Input: dimensioned drawing with shaded views. Units: mm. Origin: part minimum x, y, z. Round coordinates to 2 decimals unless told otherwise and drop trailing zeros. Loops run counter-clockwise (first coordinate to the right, second up) from the corner with the lowest first, then second, coordinate; pieces in that order, holes last. Notation, with made-up numbers: M -13.75,62.25 L 29.25,62.25 A23 ccw 29.25,99.25 Z; hole C 64.25,87 d11. An arc over 180 degrees is marked long. Write each question's results on one line, items separated by ' | '. Start each with the question number.
1. Draft query along Z for the marked faces 1, 2, 3 and 4. Return one class per face: released by +Z, released by -Z, zero draft, split by the parting line, or undercut.
2. Ray query, line 1 (Y direction, x = 4.65, z = 17.5); line 2 (Y direction, x = 4.35, z = 24); line 3 (X direction, y = 15.5, z = 9.25). Return the intervals inside material, ascending.
3. Contact query for flat-ended pins moving along their axis: pin 1 Ø7.5 at (y, z) = (12.37, 17.5) entering from -X; pin 2 Ø2 at (x, z) = (4.5, 18.5) entering from -Y; pin 3 Ø4 at (y, z) = (14.5, 23.5) entering from -X; pin 4 Ø2 at (x, z) = (1.5, 10.5) entering from +Y. Output: stop coordinate, or through.
4. Section A-A on z = 14.25. Output: boundary loops of the cut face in (x, y) (1 decimal), and give its area (3 significant figures).
5. Section C-C on x = 1.65. Output: boundary loops of the cut face in (y, z) (1 decimal).
6. Section D-D on z = 17.5. Output: boundary loops of the cut face in (x, y).
7. Section B-B on y = 11.5. Output: boundary loops of the cut face in (x, z).
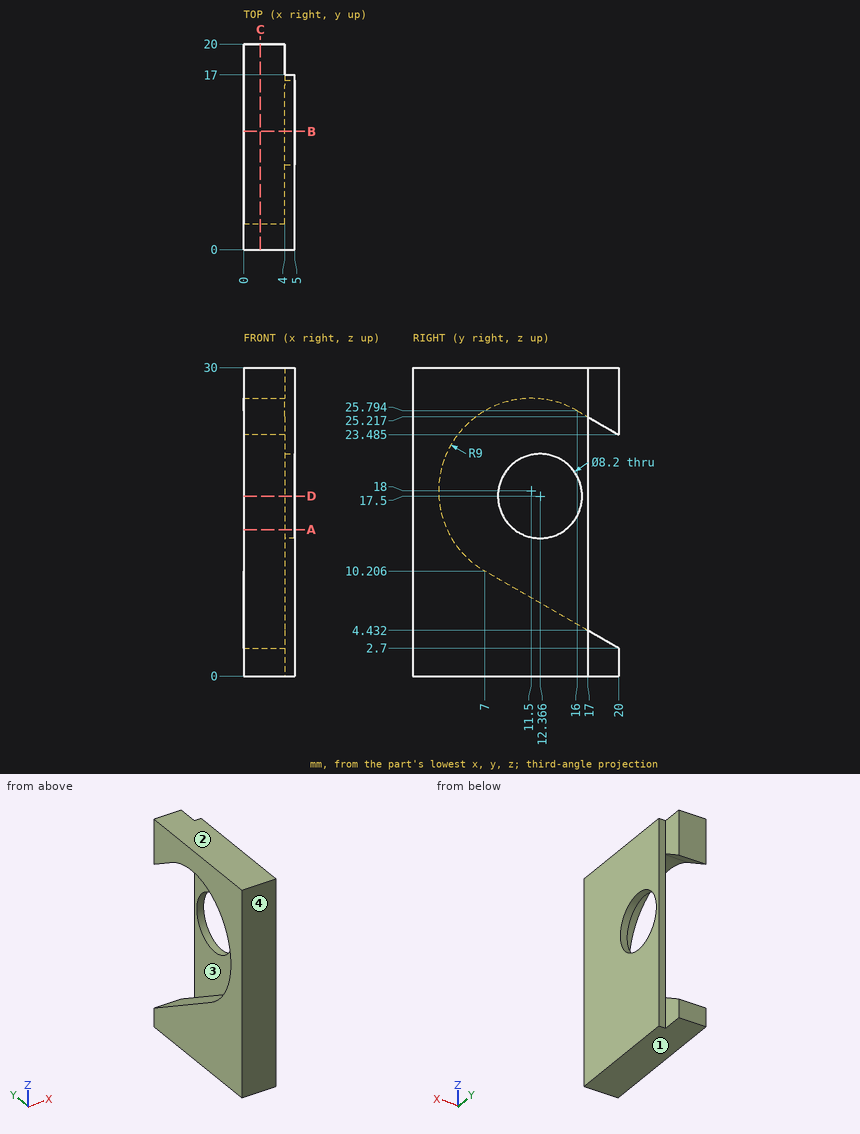
Taken from the geometry:
1) face 1: released by -Z | face 2: released by +Z | face 3: undercut | face 4: zero draft
2) line 1: 0 to 8.27, 16.47 to 17 | line 2: 0 to 17 | line 3: 4 to 5
3) pin 1: through | pin 2: y = 0 | pin 3: x = 4 | pin 4: y = 8.22
4) outline: M 0,0 L 5,0 L 5,9.9 L 4,9.9 L 4,3.3 L 0,3.3 Z; M 4,14.9 L 5,14.9 L 5,17 L 4,17 Z | area: 25.3 mm^2
5) outline: M 0,0 L 20,0 L 20,2.7 L 7,10.2 A9 cw 16,25.8 L 20,23.5 L 20,30 L 0,30 Z
6) outline: M 0,0 L 5,0 L 5,8.27 L 4,8.27 L 4,2.51 L 0,2.51 Z; M 4,16.47 L 5,16.47 L 5,17 L 4,17 Z
7) outline: M 0,0 L 5,0 L 5,13.49 L 4,13.49 L 4,7.61 L 0,7.61 Z; M 0,27 L 4,27 L 4,21.51 L 5,21.51 L 5,30 L 0,30 Z
